Answer from the drawing. Dimensions are ordinates in mm from the lowest x, y and z of the part. A direction names the side the tool comes from. Coordinates: 2 decimals unless noted, no trailing zeros. Order: outer loops, then holes, each group sorted by start corner. A loop starts at its lowest first (then second) coordinate and runs counter-clockwise, first axis right, second up. Notation, with made-up numbers: (79, -4) - (124, -4) arc R13 ccw to (124, 12) - close; hole circle Ø4 at (15.5, 87.25). An arc over 180 degrees is marked (long way). Answer as a JSON object with one key per item and string values. Group by question number.
1) Section D-D (x = 14.75) is taken. Give the vertices of the cut face in (y, z), plus the area to 3 significant figures.
2) Section B-B (y = 8.5) is taken. Give the vertices of the cut face in (x, z).
3) Section A-A (z = 14.5) is taken. Give the vertices of the cut face in (x, y), plus the area to 3 significant figures.
4) Find the intervals of material crossed by line 1 along Z through (x, y) = (5.25, 0.6); line 2 along X through (y, z) = (1, 14.25); line 3 along Y through (x, z) = (16, 1.8), in increasing order.
5) A tool of negligible diameter and unlimited length cuts with its end or side. For the marked faces 1 and 2, from which of +Z, -Z, +X, -X, +Y, -Y can it reach the whole face along a straight path? Write none if from no direction.
6) Each of these flat-tipped pins is pushed along its axis until it touches: P1, Ø3.5, axis at x = 4, y = 8.5, coming from the +Z side; P2, Ø1.5, axis at x = 3, z = 12.5, coming from the +Y side. Where does it stop, or does it pass through?
7) The mould has two halves that part along X. Classify the marked faces 3, 4, 5 and 6: released by +X, released by -X, zero draft, split by the parting line, or undercut.
8) Section C-C (z = 2.75) is taken. Give the vertices of the cut face in (x, y), plus the area to 3 significant figures.
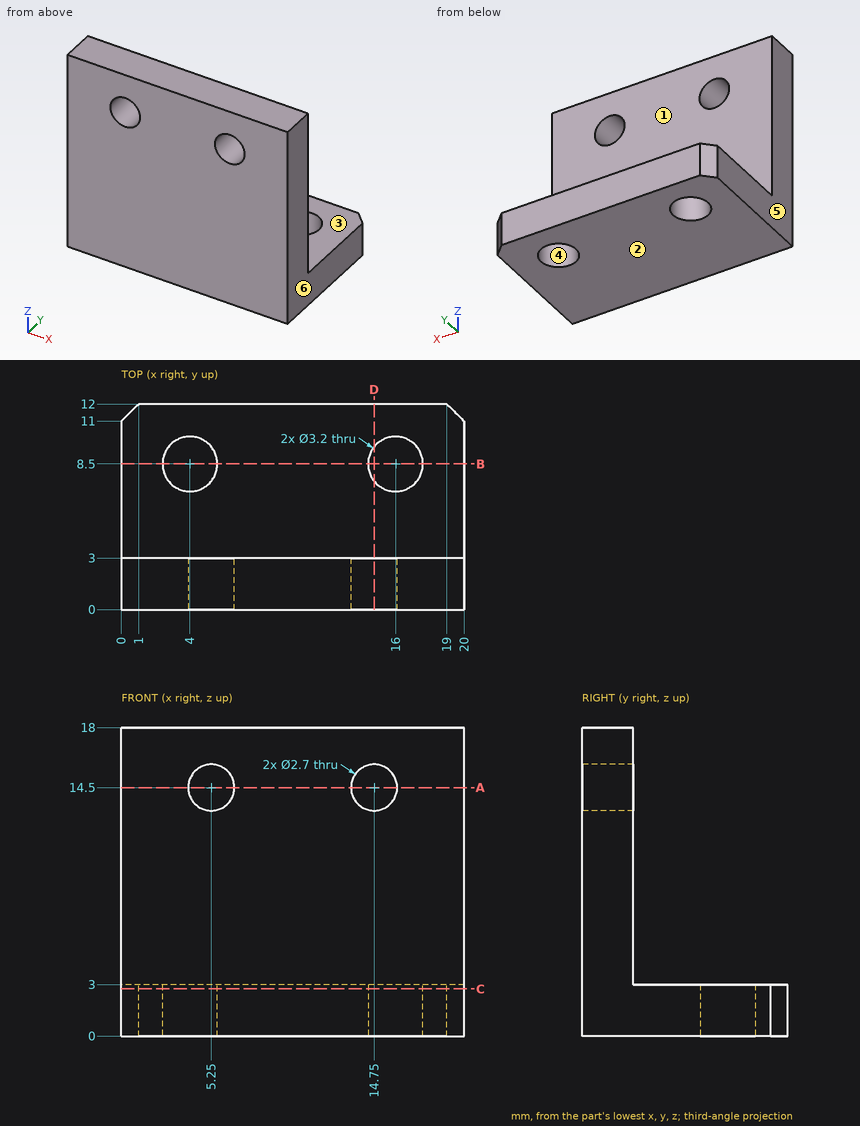
Report:
{
 "1": {"outline": "(0, 0) - (7.5, 0) - (7.5, 3) - (3, 3) - (3, 13.15) - (0, 13.15) - close; (0, 15.85) - (3, 15.85) - (3, 18) - (0, 18) - close; (9.5, 0) - (12, 0) - (12, 3) - (9.5, 3) - close", "area": "66.9 mm²"},
 "2": {"outline": "(0, 0) - (2.4, 0) - (2.4, 3) - (0, 3) - close; (5.6, 0) - (14.4, 0) - (14.4, 3) - (5.6, 3) - close; (17.6, 0) - (20, 0) - (20, 3) - (17.6, 3) - close"},
 "3": {"outline": "(0, 0) - (3.9, 0) - (3.9, 3) - (0, 3) - close; (6.6, 0) - (13.4, 0) - (13.4, 3) - (6.6, 3) - close; (16.1, 0) - (20, 0) - (20, 3) - (16.1, 3) - close", "area": "43.8 mm²"},
 "4": {"line 1": "z = 0 to 13.15, 15.85 to 18", "line 2": "x = 0 to 3.92, 6.58 to 13.42, 16.08 to 20", "line 3": "y = 0 to 6.9, 10.1 to 12"},
 "5": {"face 1": "+Z, +X, -X, +Y", "face 2": "-Z, +X, -X, +Y, -Y"},
 "6": {"P1": "stops at z = 3", "P2": "stops at y = 3"},
 "7": {"face 3": "zero draft", "face 4": "undercut", "face 5": "released by -X", "face 6": "released by +X"},
 "8": {"outline": "(0, 0) - (20, 0) - (20, 11) - (19, 12) - (1, 12) - (0, 11) - close; hole circle Ø3.2 at (4, 8.5); hole circle Ø3.2 at (16, 8.5)", "area": "223 mm²"}
}
